Verification items for this drawing (mm, ordinates from the low corner). A direction names the side the tool comes from. Coordinates: 2 decimals unless noted, no trailing zeros. Write each loop counter-clockwise with the first axis right and the second up, starting at its lowest first coordinate (ties: lowest second). Pieces come first, ordered by that corner, then holes. Notation, with made-up numbers: (84, -21) -> (134, -21) arc R22 cw to (134, 12) -> close; hole circle Ø11 at (-17.75, -26.5). An arc over 180 degrees is marked (long way). Answer as CSV lines item,"result".
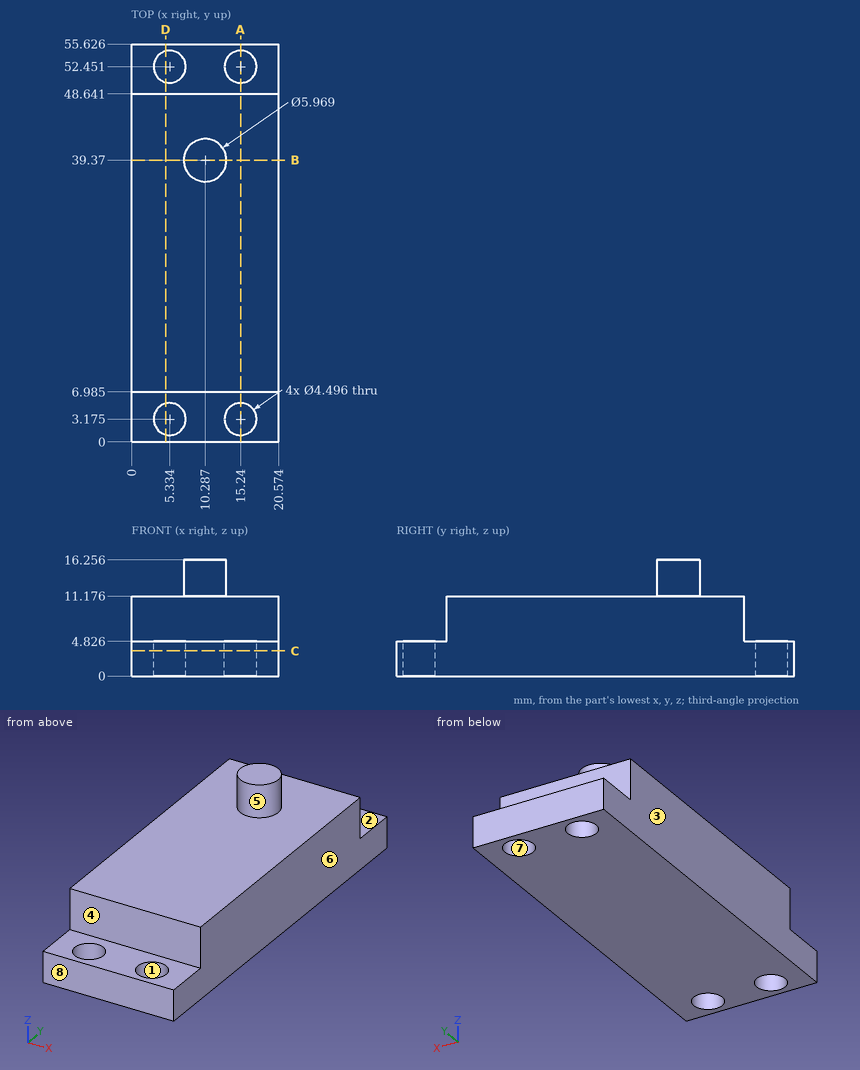
Item 1: Cross-section at C-C, the plane z = 3.5. Record the cut outline in (x, y) (1 decimal), plus the area to 3 significant figures.
Responses:
outline,"(0, 0) -> (20.6, 0) -> (20.6, 55.6) -> (0, 55.6) -> close; hole circle Ø4.5 at (5.3, 3.2); hole circle Ø4.5 at (5.3, 52.5); hole circle Ø4.5 at (15.2, 3.2); hole circle Ø4.5 at (15.2, 52.5)"
area,"1,080 mm2"
Item 2: Thickness scan on probe 1 along Y at (x, z) = (15.24, 2.35); probe 2 along X at (y, z) = (3, 1.5) (1 decimal); probe 3 along Z at (x, y) = (1.5, 5.5). Record the ranges inside material, lowest first.
Responses:
probe 1,"y = 0 to 0.93, 5.42 to 50.2, 54.7 to 55.63"
probe 2,"x = 0 to 3.1, 7.6 to 13, 17.5 to 20.6"
probe 3,"z = 0 to 4.83"
Item 3: Cross-section at D-D, the plane x = 4.75. Record the cut outline in (y, z) (1 decimal), plus the area to 3 significant figures.
Responses:
outline,"(0, 0) -> (1, 0) -> (1, 4.8) -> (0, 4.8) -> close; (5.3, 0) -> (50.3, 0) -> (50.3, 4.8) -> (48.6, 4.8) -> (48.6, 11.2) -> (7, 11.2) -> (7, 4.8) -> (5.3, 4.8) -> close; (54.6, 0) -> (55.6, 0) -> (55.6, 4.8) -> (54.6, 4.8) -> close"
area,"491 mm2"
Item 4: Depth check by flat-ended pin: pin 1 Ø10.5 at (x, y) = (9.5, 20) entering from +Z; pin 2 Ø5 at (x, y) = (15.24, 52.451) entering from +Z; pin 3 Ø5 at (x, z) = (12, 7.5) entering from +Y. Enter the tip coordinate at first touch or a pass-through.
Responses:
pin 1,"stops at z = 11.18"
pin 2,"stops at z = 4.83"
pin 3,"stops at y = 48.64"
Item 5: Cross-section at B-B, the plane y = 39.37. Record the cut outline in (x, z), plus the area to 3 significant figures.
Responses:
outline,"(0, 0) -> (20.57, 0) -> (20.57, 11.18) -> (13.27, 11.18) -> (13.27, 16.26) -> (7.3, 16.26) -> (7.3, 11.18) -> (0, 11.18) -> close"
area,"260 mm2"
Item 6: Release check for a two-part mould opening along X. For the marked faces 6, 7 and 8 record: +X half, -X half, draft (parallel to the pull), parting line (faces both ways), or undercut.
Responses:
face 6,"+X half"
face 7,"undercut"
face 8,"draft"
Item 7: Cross-section at A-A, the plane x = 15.24. Record the cut outline in (y, z) (1 decimal), plus the area to 3 significant figures.
Responses:
outline,"(0, 0) -> (0.9, 0) -> (0.9, 4.8) -> (0, 4.8) -> close; (5.4, 0) -> (50.2, 0) -> (50.2, 4.8) -> (48.6, 4.8) -> (48.6, 11.2) -> (7, 11.2) -> (7, 4.8) -> (5.4, 4.8) -> close; (54.7, 0) -> (55.6, 0) -> (55.6, 4.8) -> (54.7, 4.8) -> close"
area,"490 mm2"
Item 8: Set-up check for the marked faces 1, 2, 3, 4 and 5: record each of +Z, -Z, +X, -X, +Y, -Y from which the full face is reachable in a straight line by a thin tool's end or side.
Responses:
face 1,"+Z, -Z"
face 2,"+Z, +X, -X, +Y"
face 3,"+Z, -Z, -X, +Y, -Y"
face 4,"+Z, +X, -X, -Y"
face 5,"+Z"
